Input: part model. Units: mm. Frame: model coordinates. Give positions to 0.01 mm unless a question says otherwise; leave off trailing zeros. Order: outer loops, then holes, each group sorted by start corner. A loop starts at its lowest first (then second) coordinate and runs counter-clockwise, first axis right, second up. Notation, with made-up numbers: (-15.75, -9.75) - (1.25, -9.75) arc R20 cw to (1.25, 13.25) - close; hole circle Ø1 at (-34.5, 9). An arc over 180 degrees is marked (long way). Use a Markdown table: item, result.
from build123d import *

# Parameters (mm, degrees)
SKETCH1_R                 = 70
BOSS_EXTRUDE1_DEPTH       = 10
SKETCH2_R                 = 65
BOSS_EXTRUDE2_DEPTH       = 3
BOSS_EXTRUDE3_DEPTH       = 5
M4X0_7_TAPPED_HOLE1_D     = 3.3
M4X0_7_TAPPED_HOLE1_DEPTH = 10.1
M4X0_7_TAPPED_HOLE1_TIP   = 0.991420021
M8X1_0_TAPPED_HOLE1_D     = 7
M4X0_7_TAPPED_HOLE3_D     = 3.3
M4X0_7_TAPPED_HOLE3_DEPTH = 10.1
M4X0_7_TAPPED_HOLE3_TIP   = 0.991420021
M8X1_0_TAPPED_HOLE2_D     = 7


with BuildPart() as part:
    # Sketch1 → Boss-Extrude1 (new body)
    with BuildSketch(Plane(origin=(0, 0, 0), x_dir=(1, 0, 0), z_dir=(0, 1, 0))):
        Circle(SKETCH1_R)
    extrude(amount=BOSS_EXTRUDE1_DEPTH)

    # Sketch2 → Boss-Extrude2 (add)
    with BuildSketch(Plane.XZ):
        Circle(SKETCH2_R)
    extrude(amount=BOSS_EXTRUDE2_DEPTH)

    # Sketch3 → Boss-Extrude3 (add, symmetric)
    with BuildSketch(Plane.XY):
        with BuildLine():
            Line((-25, 55), (-25, 5))
            Line((-25, 5), (-90, 5))
            Line((-90, 5), (-112.094257771, 43.204763027))
            ThreePointArc((-112.094257771, 43.204763027), (-75.29730578, 98.944673602), (-25, 55))
        make_face()
    extrude(amount=BOSS_EXTRUDE3_DEPTH, both=True)

    # M4x0.7 Tapped Hole1
    with Locations(Plane(origin=(0, 10, 0), x_dir=(1, 0, 0), z_dir=(0, 1, 0))):
        with Locations((4, 23.622), (51.244, 23.622), (51.244, -23.622), (4, -23.622)):
            Hole(M4X0_7_TAPPED_HOLE1_D / 2, depth=M4X0_7_TAPPED_HOLE1_DEPTH)
            with Locations((0, 0, -(M4X0_7_TAPPED_HOLE1_DEPTH + M4X0_7_TAPPED_HOLE1_TIP / 2))):  # 118° drill point
                Cone(0, M4X0_7_TAPPED_HOLE1_D / 2, M4X0_7_TAPPED_HOLE1_TIP, mode=Mode.SUBTRACT)

    # M8x1.0 Tapped Hole1 (through all)
    with Locations(Plane(origin=(0, 10, 0), x_dir=(1, 0, 0), z_dir=(0, 1, 0))):
        with Locations((28.426798857, 0)):
            Hole(M8X1_0_TAPPED_HOLE1_D / 2)

    # M4x0.7 Tapped Hole3
    with Locations(Plane(origin=(-95.25342131, 45.793176502, 5), x_dir=(1, 0, 0), z_dir=(0, 0, 1))):
        with Locations((4, 23.622), (51.244, 23.622), (51.244, -23.622), (4, -23.622)):
            Hole(M4X0_7_TAPPED_HOLE3_D / 2, depth=M4X0_7_TAPPED_HOLE3_DEPTH)
            with Locations((0, 0, -(M4X0_7_TAPPED_HOLE3_DEPTH + M4X0_7_TAPPED_HOLE3_TIP / 2))):  # 118° drill point
                Cone(0, M4X0_7_TAPPED_HOLE3_D / 2, M4X0_7_TAPPED_HOLE3_TIP, mode=Mode.SUBTRACT)

    # M8x1.0 Tapped Hole2 (through all)
    with Locations(Plane(origin=(-95.25342131, 45.793176502, 5), x_dir=(1, 0, 0), z_dir=(0, 0, 1))):
        with Locations((28.426798857, 0)):
            Hole(M8X1_0_TAPPED_HOLE2_D / 2)


solid = part.part
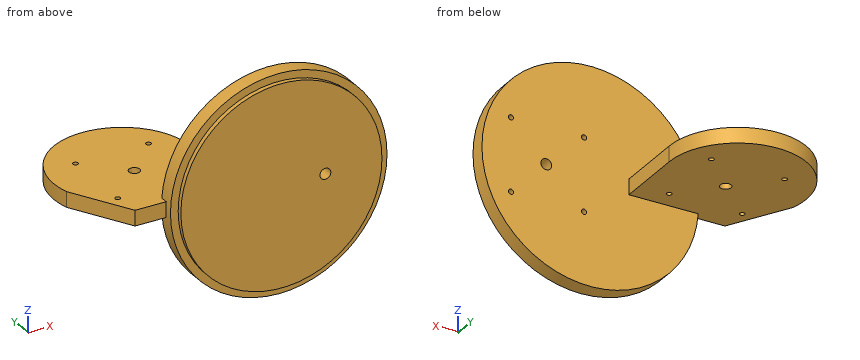
1. Section query B-B (z = 0). Return loops of the section in (x, y).
Response:
| item | result |
|---|---|
| outline | (-112.09, 43.2) - (-90, 5) - (-70, 5) - (-70, 0) - (-65, 0) - (-65, -3) - (24.93, -3) - (24.93, 10) - (-25, 10) - (-25, 55) arc R44.35 ccw (long way) to start; (31.93, -3) - (65, -3) - (65, 0) - (70, 0) - (70, 10) - (31.93, 10) - close; hole circle Ø3.3 at (-91.25, 22.17); hole circle Ø3.3 at (-91.25, 69.42); hole circle Ø7 at (-66.83, 45.79); hole circle Ø3.3 at (-44.01, 22.17); hole circle Ø3.3 at (-44.01, 69.42) |
2. Pin query (flat end, axial travel): pin 1 (2 mm diameter, centred on x = -44.01, y = 22.17, fed in from +Z); pin 2 (1 mm diameter, centred on x = -36.5, z = -50, fed in from +Y); pin 3 (3 mm diameter, centred on x = 51.244, z = -23.622, fed in from +Y); pin 4 (3 mm diameter, centred on y = 26.5, z = 0.5, fed in from +X). Return the tip coordinate at first contact, or that it passes through.
Response:
| item | result |
|---|---|
| pin 1 | passes through |
| pin 2 | stops at y = 10 |
| pin 3 | stops at y = -0.19 |
| pin 4 | stops at x = -25 |
3. Material intervals for line 1 along Z through (x, y) = (-56, 11); line 2 along Z through (x, y) = (4, 7.75); line 3 along Y through (x, z) = (37, 42.5), sorted ascending.
Response:
| item | result |
|---|---|
| line 1 | z = -5 to 5 |
| line 2 | z = -69.89 to -25.27, -21.97 to 21.97, 25.27 to 69.89 |
| line 3 | y = -3 to 10 |
4. Section query D-D (x = -54.5). Return loops of the section in (y, z), then the cut area to 3 significant figures.
Response:
| item | result |
|---|---|
| outline | (-3, -35.42) - (0, -35.42) - (0, -43.93) - (10, -43.93) - (10, -5) - (96.79, -5) - (96.79, 5) - (10, 5) - (10, 43.93) - (0, 43.93) - (0, 35.42) - (-3, 35.42) - close |
| area | 1,960 mm^2 |
5. Section query C-C (x = 0). Return loops of the section in (y, z).
Response:
| item | result |
|---|---|
| outline | (-3, -65) - (0, -65) - (0, -70) - (10, -70) - (10, 70) - (0, 70) - (0, 65) - (-3, 65) - close |
6. Section query A-A (z = 56). Return loops of the section in (x, y).
Response:
| item | result |
|---|---|
| outline | (-42, 0) - (-33, 0) - (-33, -3) - (33, -3) - (33, 0) - (42, 0) - (42, 10) - (-42, 10) - close |
